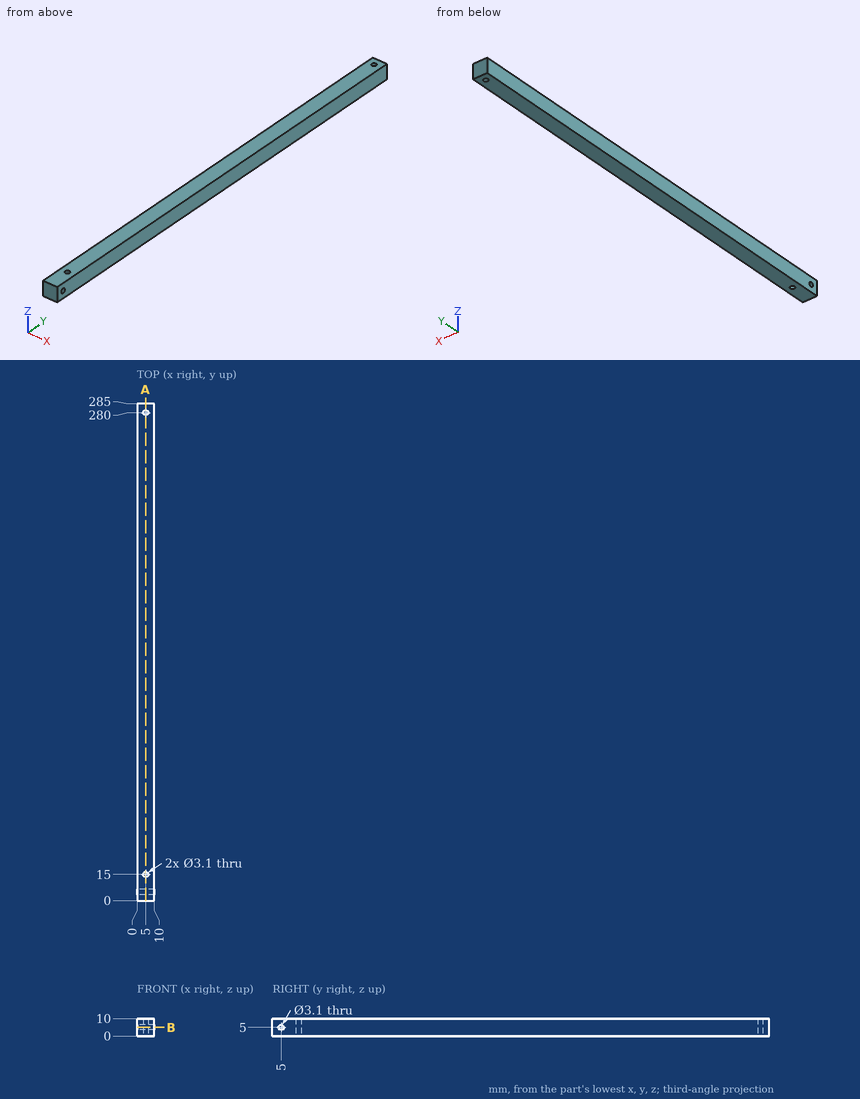
Input: dimensioned drawing with shaded views. Units: mm. Origin: part minimum x, y, z. Coordinates: 2 decimals unless noted, no trailing zeros. Write each loop counter-clockwise with the first axis right and the second up, starting at its lowest first coordinate (ties: lowest second). Pieces come first, ordered by that corner, then holes. Notation, with made-up numbers: M -40,-16 L 12,-16 A11 ccw 12,-3 Z; hole C 54,11 d8. An arc over 180 degrees is marked long. Answer as a JSON object with one key per item and string values. Group by question number.
(1) Contact query for a flat-ended pin moving along its axis: P1, Ø2.5, axis at y = 5, z = 5, coming from the -X side. Output: stop coordinate, or through.
(2) Section B-B on z = 5. Output: boundary loops of the cut face in (x, y), plus the area to 3 significant figures.
(3) Section A-A on x = 5. Output: boundary loops of the cut face in (y, z).
(4) Ray query, line 1 along Y through (x, z) = (5, 3.25); line 2 along Y through (x, z) = (6.25, 4); line 3 along X through (y, z) = (280, 8). Return the intervals inside material, ascending. Write a range as [from, to].
Result set:
{
 "1": {"P1": "passes through"},
 "2": {"outline": "M 0,0 L 10,0 L 10,3.45 L 0,3.45 Z; M 0,6.55 L 10,6.55 L 10,285 L 0,285 Z; hole C 5,15 d3.1; hole C 5,280 d3.1", "area": "2,800 mm2"},
 "3": {"outline": "M 0,0 L 13.45,0 L 13.45,10 L 0,10 Z; M 16.55,0 L 278.45,0 L 278.45,10 L 16.55,10 Z; M 281.55,0 L 285,0 L 285,10 L 281.55,10 Z; hole C 5,5 d3.1"},
 "4": {"line 1": "y = [0, 13.45], [16.55, 278.45], [281.55, 285]", "line 2": "y = [0, 3.82], [6.18, 14.08], [15.92, 279.08], [280.92, 285]", "line 3": "x = [0, 3.45], [6.55, 10]"}
}
